from build123d import *

# Parameters (mm, degrees)
SKETCH1_R           = 2.1
BOSS_EXTRUDE1_DEPTH = 40


with BuildPart() as part:
    # Sketch1 → Boss-Extrude1 (new body)
    with BuildSketch(Plane(origin=(0, 0, 0), x_dir=(-1, 0, 0), z_dir=(0, 0, -1))):
        with BuildLine():
            Line((-3.9, -0.21), (-3.9, -2.839339828))
            Line((-3.9, -2.839339828), (-6.560660172, -5.5))
            Line((-6.560660172, -5.5), (-8.2, -5.5))
            Line((-8.2, -5.5), (-8.2, -3.125))
            Line((-8.2, -3.125), (-8.545, -3.125))
            Line((-8.545, -3.125), (-10, -4.58))
            Line((-10, -4.58), (-10, -9.5))
            ThreePointArc((-10, -9.5), (-9.853553391, -9.853553391), (-9.5, -10))
            Line((-9.5, -10), (-4.58, -10))
            Line((-4.58, -10), (-3.125, -8.545))
            Line((-3.125, -8.545), (-3.125, -8.2))
            Line((-3.125, -8.2), (-5.5, -8.2))
            Line((-5.5, -8.2), (-5.5, -6.560660172))
            Line((-5.5, -6.560660172), (-2.839339828, -3.9))
            Line((-2.839339828, -3.9), (-0.21, -3.9))
            Line((-0.21, -3.9), (0, -3.69))
            Line((0, -3.69), (0.21, -3.9))
            Line((0.21, -3.9), (2.839339828, -3.9))
            Line((2.839339828, -3.9), (5.5, -6.560660172))
            Line((5.5, -6.560660172), (5.5, -8.2))
            Line((5.5, -8.2), (3.125, -8.2))
            Line((3.125, -8.2), (3.125, -8.545))
            Line((3.125, -8.545), (4.58, -10))
            Line((4.58, -10), (9.5, -10))
            ThreePointArc((9.5, -10), (9.853553391, -9.853553391), (10, -9.5))
            Line((10, -9.5), (10, -4.58))
            Line((10, -4.58), (8.545, -3.125))
            Line((8.545, -3.125), (8.2, -3.125))
            Line((8.2, -3.125), (8.2, -5.5))
            Line((8.2, -5.5), (6.560660172, -5.5))
            Line((6.560660172, -5.5), (3.9, -2.839339828))
            Line((3.9, -2.839339828), (3.9, -0.21))
            Line((3.9, -0.21), (3.69, 0))
            Line((3.69, 0), (3.9, 0.21))
            Line((3.9, 0.21), (3.9, 2.839339828))
            Line((3.9, 2.839339828), (6.560660172, 5.5))
            Line((6.560660172, 5.5), (8.2, 5.5))
            Line((8.2, 5.5), (8.2, 3.125))
            Line((8.2, 3.125), (8.545, 3.125))
            Line((8.545, 3.125), (10, 4.58))
            Line((10, 4.58), (10, 9.5))
            ThreePointArc((10, 9.5), (9.853553391, 9.853553391), (9.5, 10))
            Line((9.5, 10), (4.58, 10))
            Line((4.58, 10), (3.125, 8.545))
            Line((3.125, 8.545), (3.125, 8.2))
            Line((3.125, 8.2), (5.5, 8.2))
            Line((5.5, 8.2), (5.5, 6.560660172))
            Line((5.5, 6.560660172), (2.839339828, 3.9))
            Line((2.839339828, 3.9), (0.21, 3.9))
            Line((0.21, 3.9), (0, 3.69))
            Line((0, 3.69), (-0.21, 3.9))
            Line((-0.21, 3.9), (-2.839339828, 3.9))
            Line((-2.839339828, 3.9), (-5.5, 6.560660172))
            Line((-5.5, 6.560660172), (-5.5, 8.2))
            Line((-5.5, 8.2), (-3.125, 8.2))
            Line((-3.125, 8.2), (-3.125, 8.545))
            Line((-3.125, 8.545), (-4.58, 10))
            Line((-4.58, 10), (-9.5, 10))
            ThreePointArc((-9.5, 10), (-9.853553391, 9.853553391), (-10, 9.5))
            Line((-10, 9.5), (-10, 4.58))
            Line((-10, 4.58), (-8.545, 3.125))
            Line((-8.545, 3.125), (-8.2, 3.125))
            Line((-8.2, 3.125), (-8.2, 5.5))
            Line((-8.2, 5.5), (-6.560660172, 5.5))
            Line((-6.560660172, 5.5), (-3.9, 2.839339828))
            Line((-3.9, 2.839339828), (-3.9, 0.21))
            Line((-3.9, 0.21), (-3.69, 0))
            Line((-3.69, 0), (-3.9, -0.21))
        make_face()
        with Locations(Location((0, 0, 0), (0, 0, 180))):
            Circle(SKETCH1_R, mode=Mode.SUBTRACT)
    extrude(amount=-BOSS_EXTRUDE1_DEPTH)


solid = part.part
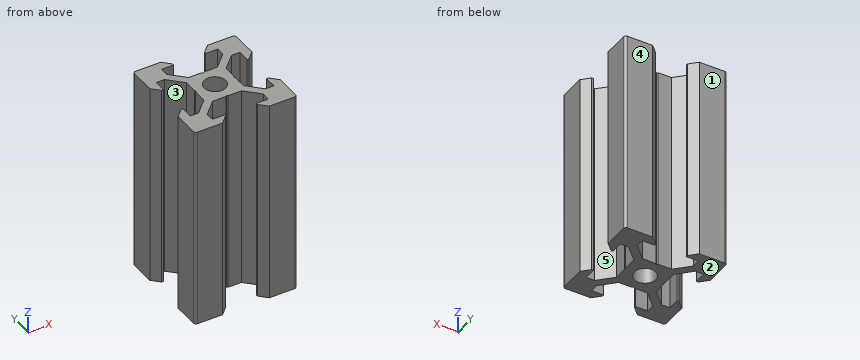
The listing builds one solid part. Answer for the finished solid, in the listing's coordinates (mm). Face numbers are marked on the shaded views. A direction names the side the tool comes from. Round coordinates to 2 decimals unless told otherwise and drop trailing zeros. Write each loop counter-clockwise with the first axis right and the second up, starting at its lowest first coordinate (ties: lowest second). Pieces come first, ordered by that corner, then holes. Notation, with made-up numbers: M -34,9.5 L -11,9.5 A22 cw -11,19.5 Z; hole C 66.25,2.25 d5. An arc over 180 degrees is marked long. Write each question's results on one line, items separated by ' | '. Start each with the question number.
Item 1: Find section B-B on x = -5. Write down the section's boundary in (y, z).
Item 2: Which of the six approach directions +Z, -Z, +X, -X, +Y, -Y give full straight-line access (tool end or side, diameter ignored) to the marked faces 4 and 5?
Item 3: Straight lines are drawn through the part: probe 1 along X at (y, z) = (-4, 27.5); probe 2 along Y at (x, z) = (-7.5, 24); probe 3 along Y at (x, z) = (-3.25, 37). For each, find the intervals that lie inside material, in ascending order.
Item 4: The mould has two halves that part along Y. Classify the marked faces 1, 2 and 3: +Y half, -Y half, draft (parallel to the pull), parting line (faces both ways), or undercut.
Item 5: Given pin 1 Ø3 at (x, z) = (3.5, 18) entering from -Y; pin 2 Ø3 at (x, z) = (-1.5, 16) entering from +Y; pin 3 Ø3 at (x, z) = (-1, 31.5) entering from +Y; pin 4 Ø4 at (x, z) = (1.5, 17.5) entering from +Y, each flat-ended and moving along its own axis, determine where each tip first touches the part or whether it passes through.
Item 6: Find section A-A on x = -7.25. Write down the section's boundary in (y, z), and give its area (3 significant figures).
Answer block:
1) outline: M -10,0 L -8.2,0 L -8.2,40 L -10,40 Z; M -6.06,0 L -3.94,0 L -3.94,40 L -6.06,40 Z; M 3.94,0 L 6.06,0 L 6.06,40 L 3.94,40 Z; M 8.2,0 L 10,0 L 10,40 L 8.2,40 Z
2) face 4: +Z, -Z, +X, -X, +Y | face 5: +Z, -Z
3) probe 1: x = -9.42 to -8.2, -5.06 to -2.94, 2.94 to 5.06, 8.2 to 9.42 | probe 2: y = -10 to -5.5, 5.5 to 10 | probe 3: y = -8.67 to -8.2, -4.31 to 4.31, 8.2 to 8.67
4) face 1: +Y half | face 2: draft | face 3: undercut
5) pin 1: stops at y = -10 | pin 2: stops at y = 4.06 | pin 3: stops at y = 3.9 | pin 4: stops at y = 8.92
6) outline: M -10,0 L -5.5,0 L -5.5,40 L -10,40 Z; M 5.5,0 L 10,0 L 10,40 L 5.5,40 Z | area: 360 mm²
